Drawing for the job (mm, zero at the part's lowest x, y, z). A direction names the side the tool comes from. Round coordinates to 2 decimals unless told otherwise and drop trailing zeros. Loops run counter-clockwise (first coordinate to the right, second up) from the corner with the lowest first, then second, coordinate; pieces in that order, holes last. Notation, with made-up numbers: M -12,8.5 L 0,8.5 A23 cw 0,31.5 Z; hole C 16,31.5 d10. An arc over 180 degrees is marked long. Answer in a Markdown table with one row per item.
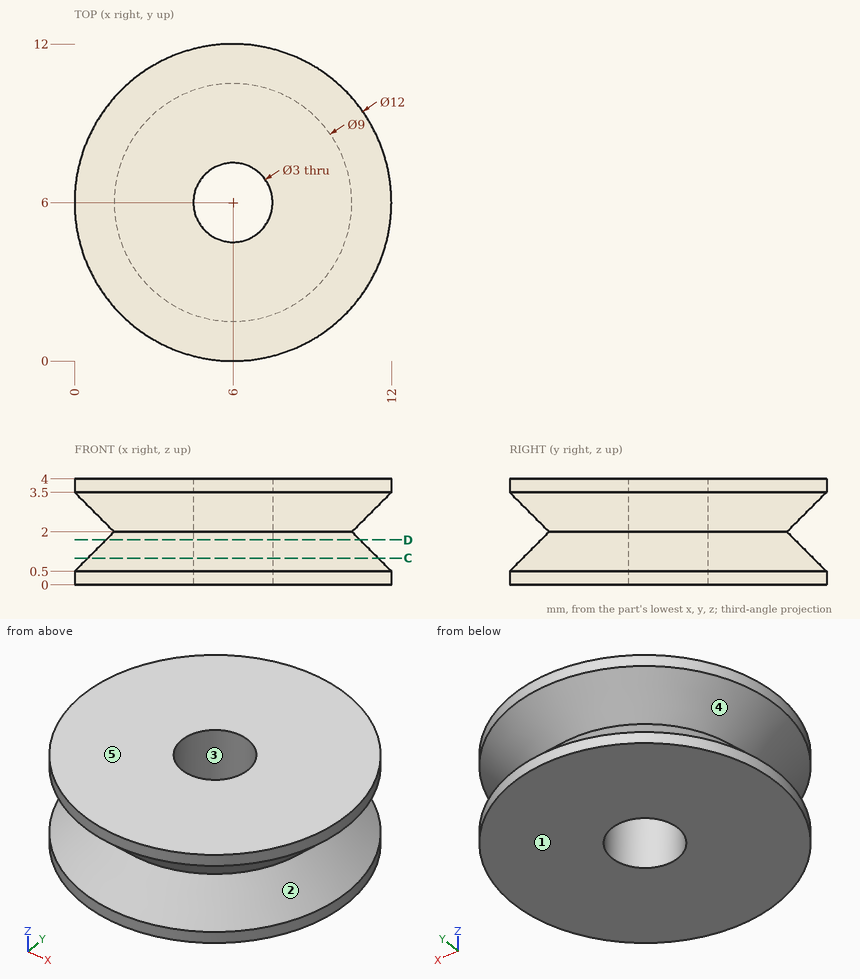
1. Saw through at C-C (z = 1). Write the cut outline in (x, y).
Verdict:
| item | result |
|---|---|
| outline | C 6,6 d11; hole C 6,6 d3 |
2. Saw through at D-D (z = 1.7). Write the cut outline in (x, y), and give its area (3 significant figures).
Verdict:
| item | result |
|---|---|
| outline | C 6,6 d9.6; hole C 6,6 d3 |
| area | 65.3 mm² |
3. Pin check, flat tip, straight feed: pin 1 (2 mm diameter, centred on x = 3.5, z = 1, fed in from +Y). Stop position of the tip, or through.
Verdict:
| item | result |
|---|---|
| pin 1 | stops at y = 11.77 |
4. Wall check: probe 1 along X at (y, z) = (7.25, 2.6) (1 decimal); probe 2 along Y at (x, z) = (6, 1.25); probe 3 along X at (y, z) = (6.25, 1.4) (1 decimal). Give the ranges that are in metal, low to high.
Verdict:
| item | result |
|---|---|
| probe 1 | x = 1.1 to 5.2, 6.8 to 10.9 |
| probe 2 | y = 0.75 to 4.5, 7.5 to 11.25 |
| probe 3 | x = 0.9 to 4.5, 7.5 to 11.1 |
5. Mould opens along Y. For the marked faces 1, 2 and 3 say: +Y half, -Y half, draft (parallel to the pull), parting line (faces both ways), or undercut.
Verdict:
| item | result |
|---|---|
| face 1 | draft |
| face 2 | parting line |
| face 3 | undercut |
6. Tool access for the marked faces 4 and 5: list every direction of +Z, -Z, +X, -X, +Y, -Y with a clear straight run to the whole face (end or side of a thin tool).
Verdict:
| item | result |
|---|---|
| face 4 | none |
| face 5 | +Z, +X, -X, +Y, -Y |
